For this review, take the finished solid that the model builds, in its own axes (mm). Face numbers are marked on the shaded views. Round coordinates to 2 decimals unless told otherwise and drop trailing zeros. Loops run counter-clockwise (first coordinate to the right, second up) from the corner with the lowest first, then second, coordinate; pieces in that order, holes last. Notation, with made-up numbers: M 69.25,34.5 L 124.25,34.5 A17 ccw 124.25,51.5 Z; hole C 42,82 d2. An arc over 180 degrees is marked long. One line per question, with ' | ' between items. Start each with the question number.
1) For probe 1 along X at (y, z) = (-20.5, 2.75); probe 2 along Y at (x, z) = (-17.5, 0.75); probe 3 along Y at (x, z) = (1, 1.25), list the stretches that pass through material, from the lowest coordinate up. Write a range as from..to.
2) Mouldability with a two-part tool opening along Y and no side actions: class the marked faces 1, 2 and 3 as pulls with the +Y half, pulls with the -Y half, needs draft (parallel to the pull), parting line crosses it, or undercut.
3) We need section A-A (x = -19.5). Give the boundary of the cut face in (y, z).
4) We need section B-B (y = -13.5). Give the boundary of the cut face in (x, z), and give its area (3 significant figures).
5) We need section C-C (z = 4.5). State how many separate pieces and enclosed holes the cut face has, and give its area (3 significant figures).
6) We need section D-D (y = 15.5). Give the boundary of the cut face in (x, z), and give its area (3 significant figures).
7) For pin 1 Ø3 at (x, z) = (15.5, 3) entering from +Y; pin 2 Ø3 at (y, z) = (17, 2.5) entering from -X; pin 3 Ø1.9 at (y, z) = (-16.5, 2) entering from +X, all flat-tipped, find the tip position at first contact; note any pin that passes through.
```python
from build123d import *

# Parameters (mm, degrees)
F0_R     = 31.75
F1_DEPTH = 6.35
F3_DEPTH = 25.4


with BuildPart() as f1:
    # F0 (on Top) → F1 (new body)
    with BuildSketch(Plane.XY):
        Circle(F0_R)
    extrude(amount=F1_DEPTH)

    # F2 (on face) → F3 (cut)
    with BuildSketch(Plane.XY.offset(6.35)):
        with BuildLine():
            Line((-1.4580238773, 3.5199810189), (0, 0))
            Line((0, 0), (0, 3.81))
            ThreePointArc((0, 3.81), (-0.7432941269, 3.7367919183), (-1.4580238773, 3.5199810189))
        make_face()
        with BuildLine():
            ThreePointArc((3.5199810189, -1.4580238773), (3.7367919183, -0.7432941269), (3.81, 0))
            Line((3.81, 0), (0, 0))
            Line((0, 0), (3.5199810189, -1.4580238773))
        make_face()
        with BuildLine():
            Line((1.4580238773, -3.5199810189), (0, 0))
            Line((0, 0), (0, -3.81))
            ThreePointArc((0, -3.81), (0.7432941269, -3.7367919183), (1.4580238773, -3.5199810189))
        make_face()
        with BuildLine():
            Line((-3.5199810189, -1.4580238773), (0, 0))
            Line((0, 0), (-3.81, 0))
            ThreePointArc((-3.81, 0), (-3.7367919183, -0.7432941269), (-3.5199810189, -1.4580238773))
        make_face()
        with BuildLine():
            Line((-3.81, 0), (0, 0))
            Line((0, 0), (-3.5199810189, 1.4580238773))
            ThreePointArc((-3.5199810189, 1.4580238773), (-3.7367919183, 0.7432941269), (-3.81, 0))
        make_face()
        with BuildLine():
            Line((0, 0), (3.81, 0))
            ThreePointArc((3.81, 0), (3.7367919183, 0.7432941269), (3.5199810189, 1.4580238773))
            Line((3.5199810189, 1.4580238773), (0, 0))
        make_face()
        with BuildLine():
            Line((0, 0), (3.5199810189, 1.4580238773))
            ThreePointArc((3.5199810189, 1.4580238773), (3.1678992229, 2.1167225878), (2.6940768363, 2.6940768363))
            Line((2.6940768363, 2.6940768363), (0, 0))
        make_face()
        with BuildLine():
            Line((1.4580238773, 3.5199810189), (0, 0))
            Line((0, 0), (2.6940768363, 2.6940768363))
            ThreePointArc((2.6940768363, 2.6940768363), (2.1167225878, 3.1678992229), (1.4580238773, 3.5199810189))
        make_face()
        with BuildLine():
            Line((0, 3.81), (0, 0))
            Line((0, 0), (1.4580238773, 3.5199810189))
            ThreePointArc((1.4580238773, 3.5199810189), (0.7432941269, 3.7367919183), (0, 3.81))
        make_face()
        with BuildLine():
            Line((-2.6940768363, 2.6940768363), (0, 0))
            Line((0, 0), (-1.4580238773, 3.5199810189))
            ThreePointArc((-1.4580238773, 3.5199810189), (-2.1167225878, 3.1678992229), (-2.6940768363, 2.6940768363))
        make_face()
        with BuildLine():
            Line((-3.5199810189, 1.4580238773), (0, 0))
            Line((0, 0), (-2.6940768363, 2.6940768363))
            ThreePointArc((-2.6940768363, 2.6940768363), (-3.1678992229, 2.1167225878), (-3.5199810189, 1.4580238773))
        make_face()
        with BuildLine():
            Line((-1.4580238773, -3.5199810189), (0, 0))
            Line((0, 0), (-2.6940768363, -2.6940768363))
            ThreePointArc((-2.6940768363, -2.6940768363), (-2.1167225878, -3.1678992229), (-1.4580238773, -3.5199810189))
        make_face()
        with BuildLine():
            Line((-2.6940768363, -2.6940768363), (0, 0))
            Line((0, 0), (-3.5199810189, -1.4580238773))
            ThreePointArc((-3.5199810189, -1.4580238773), (-3.1678992229, -2.1167225878), (-2.6940768363, -2.6940768363))
        make_face()
        with BuildLine():
            ThreePointArc((2.6940768363, -2.6940768363), (3.1678992229, -2.1167225878), (3.5199810189, -1.4580238773))
            Line((3.5199810189, -1.4580238773), (0, 0))
            Line((0, 0), (2.6940768363, -2.6940768363))
        make_face()
        with BuildLine():
            Line((2.6940768363, -2.6940768363), (0, 0))
            Line((0, 0), (1.4580238773, -3.5199810189))
            ThreePointArc((1.4580238773, -3.5199810189), (2.1167225878, -3.1678992229), (2.6940768363, -2.6940768363))
        make_face()
        with BuildLine():
            Line((0, -3.81), (0, 0))
            Line((0, 0), (-1.4580238773, -3.5199810189))
            ThreePointArc((-1.4580238773, -3.5199810189), (-0.7432941269, -3.7367919183), (0, -3.81))
        make_face()
        with BuildLine():
            ThreePointArc((-3.4020557137, 8.213289044), (-1.7343529627, 8.7191811428), (0, 8.89))
            Line((0, 8.89), (0, 25.4))
            ThreePointArc((0, 25.4), (-4.9552941792, 24.9119461222), (-9.7201591821, 23.4665401258))
            Line((-9.7201591821, 23.4665401258), (-3.4020557137, 8.213289044))
        make_face()
        with BuildLine():
            ThreePointArc((3.4020557137, 8.213289044), (4.9390193715, 7.3917648534), (6.2861792847, 6.2861792847))
            Line((6.2861792847, 6.2861792847), (17.9605122421, 17.9605122421))
            ThreePointArc((17.9605122421, 17.9605122421), (14.1114839187, 21.1193281525), (9.7201591821, 23.4665401258))
            Line((9.7201591821, 23.4665401258), (3.4020557137, 8.213289044))
        make_face()
        with BuildLine():
            ThreePointArc((8.213289044, 3.4020557137), (8.7191811428, 1.7343529627), (8.89, 0))
            Line((8.89, 0), (25.4, 0))
            ThreePointArc((25.4, 0), (24.9119461222, 4.9552941792), (23.4665401258, 9.7201591821))
            Line((23.4665401258, 9.7201591821), (8.213289044, 3.4020557137))
        make_face()
        with BuildLine():
            Line((23.4665401258, -9.7201591821), (8.213289044, -3.4020557137))
            ThreePointArc((8.213289044, -3.4020557137), (7.3917648534, -4.9390193715), (6.2861792847, -6.2861792847))
            Line((6.2861792847, -6.2861792847), (17.9605122421, -17.9605122421))
            ThreePointArc((17.9605122421, -17.9605122421), (21.1193281525, -14.1114839187), (23.4665401258, -9.7201591821))
        make_face()
        with BuildLine():
            ThreePointArc((3.4020557137, -8.213289044), (1.7343529627, -8.7191811428), (0, -8.89))
            Line((0, -8.89), (0, -25.4))
            ThreePointArc((0, -25.4), (4.9552941792, -24.9119461222), (9.7201591821, -23.4665401258))
            Line((9.7201591821, -23.4665401258), (3.4020557137, -8.213289044))
        make_face()
        with BuildLine():
            ThreePointArc((-3.4020557137, -8.213289044), (-4.9390193715, -7.3917648534), (-6.2861792847, -6.2861792847))
            Line((-6.2861792847, -6.2861792847), (-17.9605122421, -17.9605122421))
            ThreePointArc((-17.9605122421, -17.9605122421), (-14.1114839187, -21.1193281525), (-9.7201591821, -23.4665401258))
            Line((-9.7201591821, -23.4665401258), (-3.4020557137, -8.213289044))
        make_face()
        with BuildLine():
            ThreePointArc((-8.213289044, -3.4020557137), (-8.7191811428, -1.7343529627), (-8.89, 0))
            Line((-8.89, 0), (-25.4, 0))
            ThreePointArc((-25.4, 0), (-24.9119461222, -4.9552941792), (-23.4665401258, -9.7201591821))
            Line((-23.4665401258, -9.7201591821), (-8.213289044, -3.4020557137))
        make_face()
        with BuildLine():
            ThreePointArc((-8.213289044, 3.4020557137), (-7.3917648534, 4.9390193715), (-6.2861792847, 6.2861792847))
            Line((-6.2861792847, 6.2861792847), (-17.9605122421, 17.9605122421))
            ThreePointArc((-17.9605122421, 17.9605122421), (-21.1193281525, 14.1114839187), (-23.4665401258, 9.7201591821))
            Line((-23.4665401258, 9.7201591821), (-8.213289044, 3.4020557137))
        make_face()
    extrude(amount=-F3_DEPTH, mode=Mode.SUBTRACT)


solid = f1.part
```
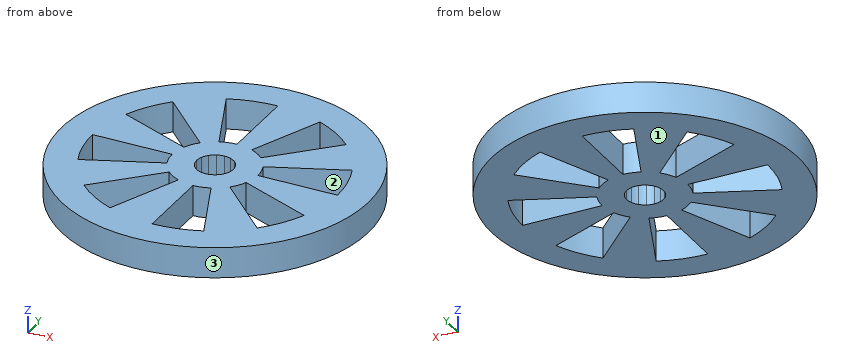
Answers below:
1) probe 1: -24.24..-15, -8.49..0, 8.49..24.24 | probe 2: -26.49..-18.41, -17.5..-7.25, 0..7.25, 17.5..26.49 | probe 3: -31.73..-25.38, -8.83..-3.68, 3.68..31.73
2) face 1: needs draft | face 2: undercut | face 3: parting line crosses it
3) outline: M -25.06,0 L -8.08,0 L -8.08,6.35 L -25.06,6.35 Z; M 0,0 L 8.08,0 L 8.08,6.35 L 0,6.35 Z; M 16.28,0 L 25.06,0 L 25.06,6.35 L 16.28,6.35 Z
4) outline: M -28.74,0 L -13.5,0 L -13.5,6.35 L -28.74,6.35 Z; M -5.59,0 L 0,0 L 0,6.35 L -5.59,6.35 Z; M 5.59,0 L 13.5,0 L 13.5,6.35 L 5.59,6.35 Z; M 21.52,0 L 28.74,0 L 28.74,6.35 L 21.52,6.35 Z | area: 228 mm^2
5) separate pieces: 1 | enclosed holes: 9 | area: 2,230 mm^2
6) outline: M -27.71,0 L -20.12,0 L -20.12,6.35 L -27.71,6.35 Z; M -15.5,0 L -6.42,0 L -6.42,6.35 L -15.5,6.35 Z; M 0,0 L 6.42,0 L 6.42,6.35 L 0,6.35 Z; M 15.5,0 L 27.71,0 L 27.71,6.35 L 15.5,6.35 Z | area: 224 mm^2
7) pin 1: y = 28.5 | pin 2: x = -27.71 | pin 3: x = 27.68
